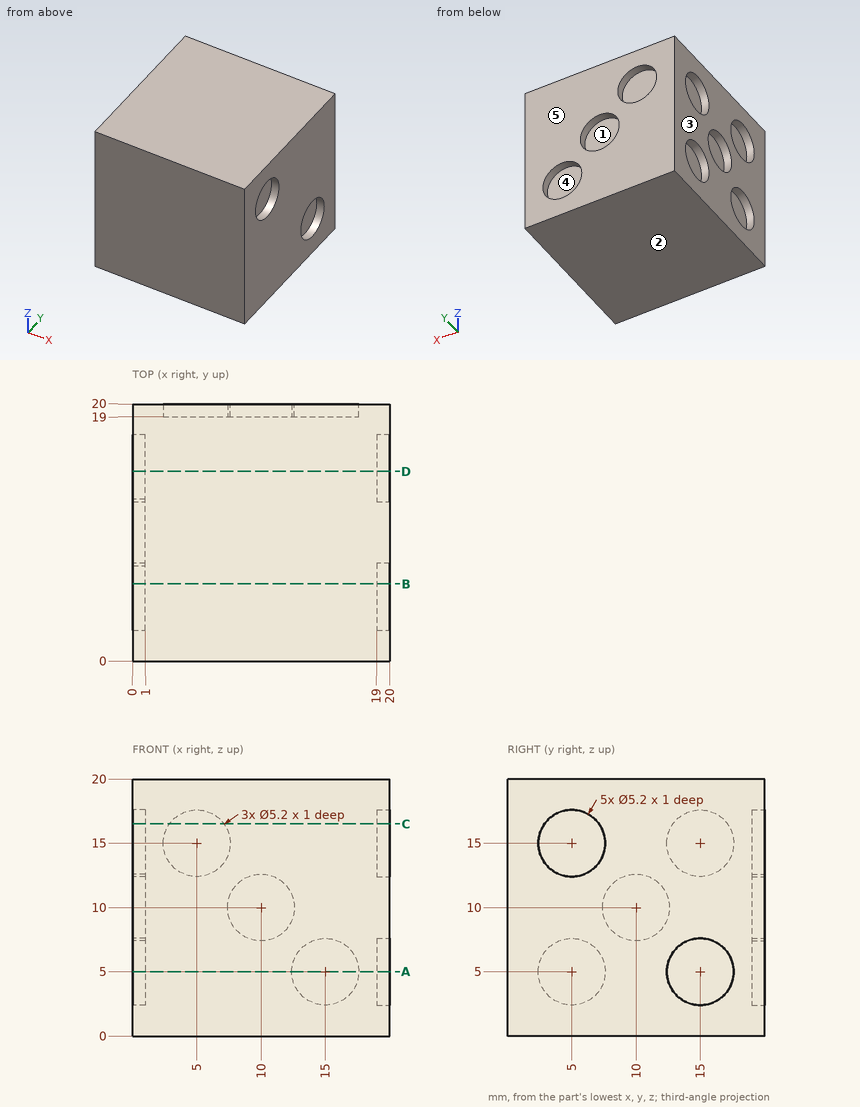
Job drawing, mm, ordinate dimensions from the low corner. One solid piece. A direction names the side the tool comes from. Give positions to 0.01 mm unless a question says otherwise; leave off trailing zeros. Write each loop counter-clockwise with the first axis right and the second up, starting at its lowest first coordinate (ties: lowest second). Pieces come first, ordered by that corner, then holes. Notation, with made-up numbers: (-23.75, 19.5) - (22.25, 19.5) arc R15 cw to (22.25, 38.5) - close; hole circle Ø11 at (9, 80.25). An arc over 180 degrees is marked (long way). Answer as CSV lines item,"result".
1. Band-saw the part on C-C (z = 16.5). Write the cut outline in (x, y), and give its area (3 significant figures).
Responses:
outline,"(0, 0) - (20, 0) - (20, 2.88) - (19, 2.88) - (19, 7.12) - (20, 7.12) - (20, 20) - (7.12, 20) - (7.12, 19) - (2.88, 19) - (2.88, 20) - (0, 20) - (0, 17.12) - (1, 17.12) - (1, 12.88) - (0, 12.88) - (0, 7.12) - (1, 7.12) - (1, 2.88) - (0, 2.88) - close"
area,"383 mm2"
2. Pin check, flat tip, straight feed: pin 1 (4 mm diameter, centred on y = 5, z = 15, fed in from -X). Stop position of the tip, or through.
Responses:
pin 1,"stops at x = 1"
3. Drill centre lines: L1, parallel to Z at x = 0.55, y = 5; L2, parallel to Z at x = 10, y = 19.6; L3, parallel to Z at x = 19.5, y = 15. Where is each one in solid material? Low to high. Write a range as [from, to].
Responses:
L1,"z = [0, 2.4], [7.6, 12.4], [17.6, 20]"
L2,"z = [0, 7.4], [12.6, 20]"
L3,"z = [0, 2.4], [7.6, 20]"
4. Band-saw the part on D-D (y = 14.75). Write the cut outline in (x, z), and give its area (3 significant figures).
Responses:
outline,"(0, 0) - (20, 0) - (20, 2.41) - (19, 2.41) - (19, 7.59) - (20, 7.59) - (20, 20) - (0, 20) - (0, 17.59) - (1, 17.59) - (1, 12.41) - (0, 12.41) - (0, 7.59) - (1, 7.59) - (1, 2.41) - (0, 2.41) - close"
area,"384 mm2"
5. Band-saw the part on B-B (y = 6). Write the cut outline in (x, z), and give its area (3 significant figures).
Responses:
outline,"(0, 0) - (20, 0) - (20, 12.6) - (19, 12.6) - (19, 17.4) - (20, 17.4) - (20, 20) - (0, 20) - (0, 17.4) - (1, 17.4) - (1, 12.6) - (0, 12.6) - (0, 7.4) - (1, 7.4) - (1, 2.6) - (0, 2.6) - close"
area,"386 mm2"
6. Band-saw the part on A-A (z = 5). Write the cut outline in (x, y).
Responses:
outline,"(0, 0) - (20, 0) - (20, 12.4) - (19, 12.4) - (19, 17.6) - (20, 17.6) - (20, 20) - (17.6, 20) - (17.6, 19) - (12.4, 19) - (12.4, 20) - (0, 20) - (0, 17.6) - (1, 17.6) - (1, 12.4) - (0, 12.4) - (0, 7.6) - (1, 7.6) - (1, 2.4) - (0, 2.4) - close"
7. 3-axis set-ups, long thin cutter, end or side, ignore diameter. For the marked faces 4 and 5: which of +Z, -Z, +X, -X, +Y, -Y reach the whole face in a straight line?
Responses:
face 4,"+Y"
face 5,"+Z, -Z, +X, -X, +Y"
8. Two-plate mould, pull along Z, no slides. Class the marked faces 1, 2 and 3: +Z half, -Z half, draft (parallel to the pull), parting line (faces both ways), or undercut.
Responses:
face 1,"undercut"
face 2,"-Z half"
face 3,"draft"
